The figure shows three views and two pictorial views of one solid part (mm, origin at its lowest corner). Answer the questions. A direction names the side the tool comes from. Give positions to 0.01 mm unless a question says otherwise; leave off trailing zeros. Write each loop counter-clockwise with the first axis right and the second up, starting at its lowest first coordinate (ties: lowest second). Pieces come first, ordered by that corner, then holes. Notation, with made-up numbers: (51.25, 89.5) -> (110.25, 89.5) arc R19 cw to (110.25, 109.5) -> close; hole circle Ø5 at (89, 55). An arc over 180 degrees is marked (long way). Write each question's results on one line, items separated by ' | '. Start each with the question number.
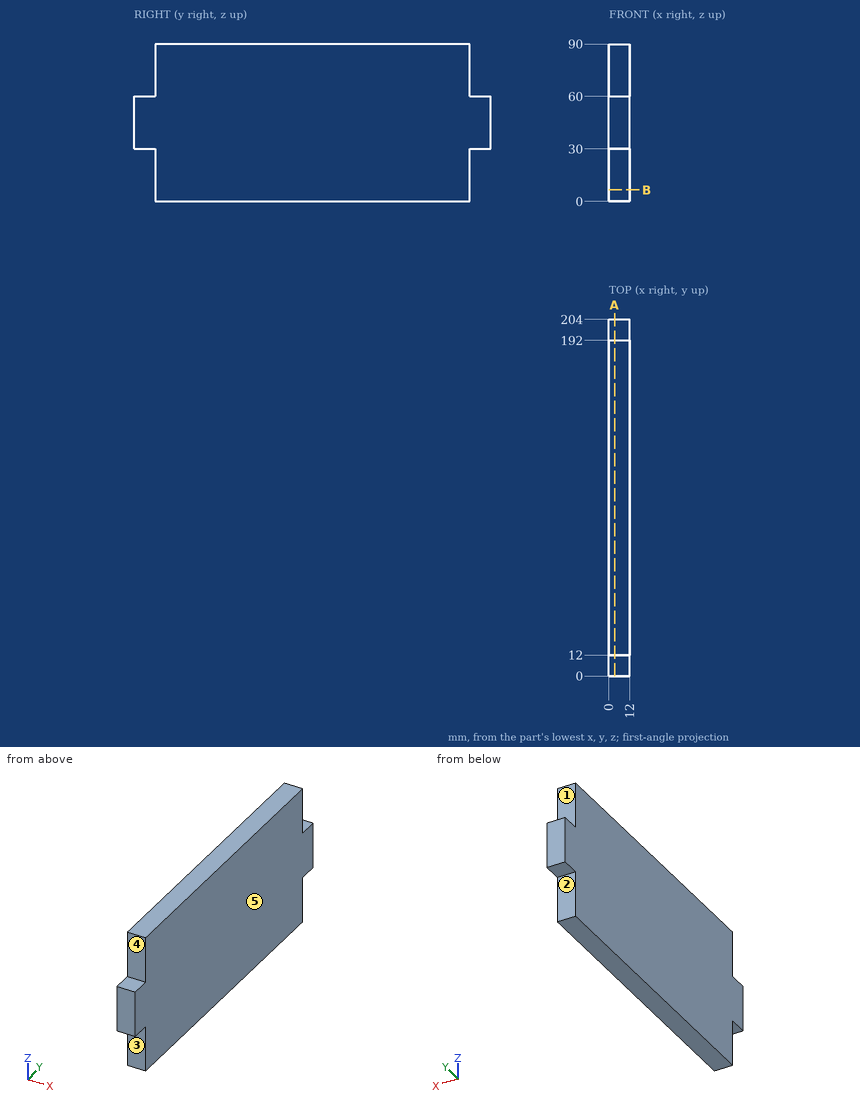
1. Consider probe 1 along Y at (x, z) = (10, 63). Determine where the line is inside the solid, lowest interval first. Write a range as [from, to].
2. Section A-A (x = 3.25) is taken. Write down the section's boundary in (y, z), then the cut area to 3 significant figures.
3. A tool of negligible diameter and unlimited length cuts with its end or side. For the marked faces 1, 2, 3, 4 and 5, from which of +Z, -Z, +X, -X, +Y, -Y can it reach the whole face along a straight path? Write none if from no direction.
4. Each of these flat-tipped pins is pushed along its axis until it touches: pin 1 Ø10 at (y, z) = (118.5, 15.5) entering from -X; pin 2 Ø6 at (x, y) = (6.5, 5.5) entering from +Z; pin 3 Ø3.5 at (x, z) = (6.5, 13.5) entering from -Y; pin 4 Ø6 at (x, z) = (5, 70) entering from +Y. Where does it stop, or does it pass through?
5. Section B-B (z = 6.5) is taken. Write down the section's boundary in (x, y).
Results:
1) probe 1: y = [12, 192]
2) outline: (0, 30) -> (12, 30) -> (12, 0) -> (192, 0) -> (192, 30) -> (204, 30) -> (204, 60) -> (192, 60) -> (192, 90) -> (12, 90) -> (12, 60) -> (0, 60) -> close | area: 16,900 mm²
3) face 1: +Z, +X, -X, +Y | face 2: -Z, +X, -X, +Y | face 3: -Z, +X, -X, -Y | face 4: +Z, +X, -X, -Y | face 5: +Z, -Z, +X, +Y, -Y
4) pin 1: stops at x = 0 | pin 2: stops at z = 60 | pin 3: stops at y = 12 | pin 4: stops at y = 192
5) outline: (0, 12) -> (12, 12) -> (12, 192) -> (0, 192) -> close
